The model under review builds one solid part; all positions refer to its coordinate system, in mm. Face numbers are marked on the shaded views. A direction names the side the tool comes from. Round coordinates to 2 decimals unless told otherwise and drop trailing zeros. Order: outer loops, then holes, each group sorted by start corner. A loop starts at its lowest first (then second) coordinate and runs counter-clockwise, first axis right, second up.
from build123d import *

# Parameters (mm, degrees)
EXTRUDE_1_DEPTH     = 136
SKETCH_3_R          = 1.5
CUT_EXTRUDE_1_DEPTH = 136
SKETCH_4_R          = 2.5
CUT_EXTRUDE_2_DEPTH = 136
CUT_EXTRUDE_3_DEPTH = 136


with BuildPart() as part:
    # 草图2 → 凸台-拉伸1 (new body)
    with BuildSketch(Plane.XY):
        Polygon((-38.864866985, -21.515849201), (-38.864866985, 58.484150799), (-21.335725209, 82.830181043), (-17.335725209, 82.830181043), (-34.864866985, 58.484150799), (-34.864866985, -21.515849201), align=None)
    extrude(amount=EXTRUDE_1_DEPTH)

    # 草图3 → 切除-拉伸1 (cut)
    with BuildSketch(Plane(origin=(-34.864866985, 0, 0), x_dir=(0, 0, -1), z_dir=(1, 0, 0))):
        with Locations(Location((-131, 40.484150799, 0), (0, 0, 90))):
            Circle(SKETCH_3_R)
        with Locations(Location((-131, -9.515849201, 0), (0, 0, 90))):
            Circle(SKETCH_3_R)
        with Locations(Location((-5, 40.484150799, 0), (0, 0, 90))):
            Circle(SKETCH_3_R)
        with Locations(Location((-5, -9.515849201, 0), (0, 0, 90))):
            Circle(SKETCH_3_R)
    extrude(amount=-CUT_EXTRUDE_1_DEPTH, mode=Mode.SUBTRACT)

    # 草图4 → 切除-拉伸2 (cut)
    with BuildSketch(Plane(origin=(-50.693793177, 36.499531087, 0), x_dir=(0, 0, -1), z_dir=(0.8115343414514944, -0.5843047258450759, 0))):
        with Locations(Location((-125, 45.090190259, 0), (0, 0, 90))):
            Circle(SKETCH_4_R)
        with Locations(Location((-11, 45.090190259, 0), (0, 0, 90))):
            Circle(SKETCH_4_R)
    extrude(amount=-CUT_EXTRUDE_2_DEPTH, mode=Mode.SUBTRACT)

    # 草图5 → 切除-拉伸3 (cut)
    with BuildSketch(Plane(origin=(-50.693793177, 36.499531087, 0), x_dir=(0, 0, -1), z_dir=(0.8115343414514944, -0.5843047258450759, 0))):
        Polygon((-136, 44.378333204), (-136, 60.422396469), (-128.660805907, 57.090190259), align=None)
        Polygon((-7.339194093, 57.090190259), (0, 57.090190259), (0, 44.378333204), align=None)
    extrude(amount=-CUT_EXTRUDE_3_DEPTH, mode=Mode.SUBTRACT)


solid = part.part
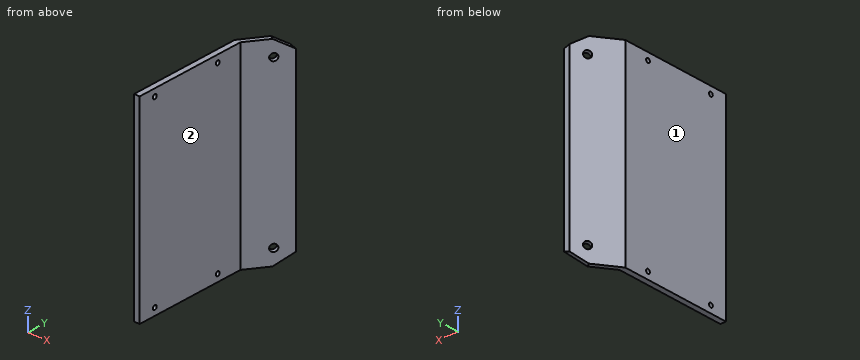
(1) To check wall thickness, follow L1, parallel to X at y = 7, z = 7.5; L2, parallel to Y at x = -26.25, z = 125.5; L3, parallel to Y at x = -18.75, z = 114. State the ranges of each line that lie inside material, in increasing order.
(2) Tool access review of the marked faces 1 and 2: name each direction out of +Z, -Z, +X, -X, +Y, -Y from which nothing blocks a thin tool from reaching the whole face with its end or side.
(3) We need section C-C (x = -30). Give the boundary of the cut face in (y, z), and give its area (3 significant figures).
(4) We need section A-A (z = 106.5). Give the boundary of the cut face in (x, y), and give its area (3 significant figures).
(5) Clearance check with flat-ended pins moving along their axes: P1, Ø4, axis at y = 40.48, z = 5, coming from the +X side; P2, Ø1.5, axis at x = -23.5, z = 110, coming from the +Y side; P3, Ø1, axis at y = 59.5, z = 106, coming from the -X side. State where each tip first meets the part, or that it passes through.
(6) We need section B-B (y = 2). Give the boundary of the cut face in (x, z).
Verdict:
1. L1: x = -38.86 to -34.86
1. L2: y = 70.45 to 71.44
1. L3: y = 80.87 to 82.83
2. face 1: +Z, -Z, -X, +Y, -Y
2. face 2: +Z, -Z, +X, -Y
3. outline: (65.24, 0) - (70.8, 0) - (70.8, 136) - (65.24, 136) - close
3. area: 756 mm2
4. outline: (-38.86, -21.52) - (-34.86, -21.52) - (-34.86, 58.48) - (-17.34, 82.83) - (-21.34, 82.83) - (-38.86, 58.48) - close
4. area: 417 mm2
5. P1: stops at x = -34.86
5. P2: stops at y = 80.87
5. P3: stops at x = -38.49
6. outline: (-38.86, 0) - (-34.86, 0) - (-34.86, 136) - (-38.86, 136) - close
